Work out the finished part from the listing and answer in its coordinate system (mm). Face numbers are marked on the shaded views. A direction names the side the tool comes from. Give positions to 0.01 mm unless a question says otherwise; leave off trailing zeros. Loops run counter-clockwise (first coordinate to the right, second up) from the corner with the lowest first, then second, coordinate; pieces in that order, holes last.
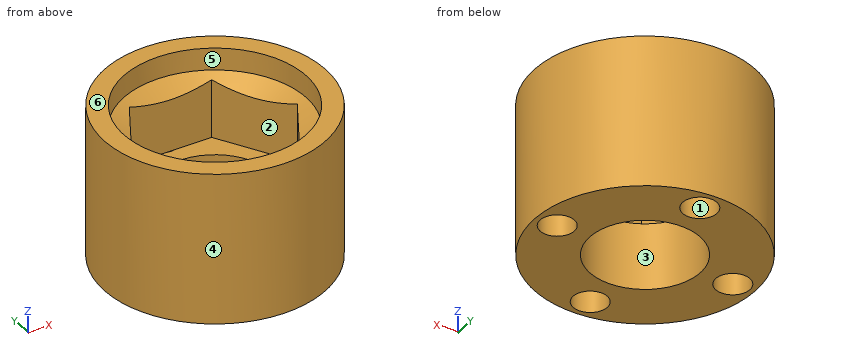
```python
from build123d import *

# Parameters (mm, degrees)
F0_R     = 10
F1_DEPTH = 13.7
F3_DEPTH = 7.7
F5_R     = 1.55
F6_DEPTH = 6
F8_R     = 5
F9_DEPTH = 25


with BuildPart() as f1:
    # F0 (on Top) → F1 (new body)
    with BuildSketch(Plane.XY):
        Circle(F0_R)
    extrude(amount=F1_DEPTH)

    # F2 (on face) → F3 (cut)
    with BuildSketch(Plane.XY.offset(13.7)):
        Polygon((3.752777, 6.5), (-3.752777, 6.5), (-7.505553, 0), (-3.752777, -6.5), (3.752777, -6.5), (7.505553, 0), align=None)
    extrude(amount=-F3_DEPTH, mode=Mode.SUBTRACT)

    # F5 (on face) → F6 (cut)
    with BuildSketch(Plane(origin=(0, 0, 0), x_dir=(1, 0, 0), z_dir=(0, 0, -1))):
        with Locations((0, 8)):
            Circle(F5_R)
        with Locations((0, -8)):
            Circle(F5_R)
        with Locations((8, 0)):
            Circle(F5_R)
        with Locations((-8, 0)):
            Circle(F5_R)
    extrude(amount=-F6_DEPTH, mode=Mode.SUBTRACT)

    # F4 (on Right) → F7 (revolve, cut)
    with BuildSketch(Plane.YZ):
        Polygon((8.25, 13.7), (0, 13.7), (0, 10.7), (6.5, 10.7), (8.25, 11.7), align=None)
    revolve(axis=Axis((0, 0, 12.2), (0, 0, 1)), mode=Mode.SUBTRACT)

    # F8 (on face) → F9 (cut)
    with BuildSketch(Plane(origin=(0, 0, 0), x_dir=(1, 0, 0), z_dir=(0, 0, -1))):
        Circle(F8_R)
    extrude(amount=-F9_DEPTH, mode=Mode.SUBTRACT)


solid = f1.part
```
Q1. Determine the mould class of the marked faces 4, 5 and 6 for opening direction Y: +Y half, -Y half, draft (parallel to the pull), parting line (faces both ways), or undercut.
Q2. Section C-C on z = 11 is taken. Give the vertices of the cut face in (x, y) (3 decimals).
Q3. Section B-B on z = 6.5 is taken. Give the vertices of the cut face in (x, y), plus the area to 3 significant figures.
Q4. Given pin 1 (1.6 mm diameter, centred on x = 1, z = 8, fed in from -Y); pin 2 (5 mm diameter, centred on x = -3.5, z = 2.5, fed in from -Y); pin 3 (4 mm diameter, centred on x = 2.5, y = -3, fed in from +Z), each flat-ended and moving along its own axis, determine where each tip first touches the part or whether it passes through.
Q5. Section A-A on x = 0 is taken. Give the vertices of the cut face in (y, z).
Q6. Consider line 1 along Y through (x, z) = (0, 2.15); line 2 along Y through (x, z) = (-0.75, 1); line 3 along Y through (x, z) = (-8, 4.65). Determine where each line is inside the solid, lowest interval first.
Q7. Which of the six approach directions +Z, -Z, +X, -X, +Y, -Y give full straight-line access (tool end or side, diameter ignored) to the marked faces 1, 2 and 3?
Check result:
1. face 4: parting line
1. face 5: undercut
1. face 6: draft
2. outline: circle Ø20 at (0, 0); hole (-7.506, 0) - (-6.962, -0.942) arc R7.025 ccw to (-4.297, -5.558) - (-3.753, -6.5) - (-2.665, -6.5) arc R7.025 ccw to (2.665, -6.5) - (3.753, -6.5) - (4.297, -5.558) arc R7.025 ccw to (6.962, -0.942) - (7.506, 0) - (6.962, 0.942) arc R7.025 ccw to (4.297, 5.558) - (3.753, 6.5) - (2.665, 6.5) arc R7.025 ccw to (-2.665, 6.5) - (-3.753, 6.5) - (-4.297, 5.558) arc R7.025 ccw to (-6.962, 0.942) - close
3. outline: circle Ø20 at (0, 0); hole (-7.51, 0) - (-3.75, -6.5) - (3.75, -6.5) - (7.51, 0) - (3.75, 6.5) - (-3.75, 6.5) - close
3. area: 168 mm2
4. pin 1: stops at y = -10
4. pin 2: stops at y = -9.95
4. pin 3: stops at z = 6
5. outline: (-10, 0) - (-9.55, 0) - (-9.55, 6) - (-6.5, 6) - (-6.5, 10.7) - (-8.25, 11.7) - (-8.25, 13.7) - (-10, 13.7) - close; (-6.45, 0) - (-5, 0) - (-5, 6) - (-6.45, 6) - close; (5, 0) - (6.45, 0) - (6.45, 6) - (5, 6) - close; (6.5, 6) - (9.55, 6) - (9.55, 0) - (10, 0) - (10, 13.7) - (8.25, 13.7) - (8.25, 11.7) - (6.5, 10.7) - close
6. line 1: y = -10 to -9.55, -6.45 to -5, 5 to 6.45, 9.55 to 10
6. line 2: y = -9.97 to -9.36, -6.64 to -4.94, 4.94 to 6.64, 9.36 to 9.97
6. line 3: y = -6 to -1.55, 1.55 to 6
7. face 1: -Z
7. face 2: +Z
7. face 3: +Z, -Z
